from build123d import *

# Parameters (mm, degrees)
ESQUISSE1_R             = 16
BOSS_EXTRU_2_DEPTH      = 30
ESQUISSE2_R             = 18.5
BOSS_EXTRU_3_DEPTH      = 25
ESQUISSE3_R             = 1
ENL_V_MAT_EXTRU_1_DEPTH = 3.5
ESQUISSE5_R             = 6
BOSS_EXTRU_4_DEPTH      = 6
ESQUISSE6_R             = 3
BOSS_EXTRU_5_DEPTH      = 15.5
ESQUISSE7_W             = 7.308646468
ESQUISSE7_H             = 1
ENL_V_MAT_EXTRU_2_DEPTH = 12


with BuildPart() as part:
    # Esquisse1 → Boss.-Extru.2 (new body)
    with BuildSketch(Plane.XY):
        Circle(ESQUISSE1_R)
    extrude(amount=BOSS_EXTRU_2_DEPTH)

    # Esquisse2 → Boss.-Extru.3 (add)
    with BuildSketch(Plane.XY.offset(30)):
        Circle(ESQUISSE2_R)
    extrude(amount=BOSS_EXTRU_3_DEPTH)

    # Esquisse3 → Enlèv. mat.-Extru.1 (cut)
    with BuildSketch(Plane.XY.offset(55)):
        with Locations(Location((-15.5, 0, 0), (0, 0, 180))):
            Circle(ESQUISSE3_R)
        with Locations(Location((7.75, -13.423393759, 0), (0, 0, 180))):
            Circle(ESQUISSE3_R)
        with Locations(Location((15.5, 0, 0), (0, 0, 180))):
            Circle(ESQUISSE3_R)
        with Locations(Location((7.75, 13.423393759, 0), (0, 0, 180))):
            Circle(ESQUISSE3_R)
    extrude(amount=-ENL_V_MAT_EXTRU_1_DEPTH, mode=Mode.SUBTRACT)

    # Esquisse5 → Boss.-Extru.4 (add)
    with BuildSketch(Plane.XY.offset(55)):
        with Locations((0, 7)):
            Circle(ESQUISSE5_R)
    extrude(amount=BOSS_EXTRU_4_DEPTH)

    # Esquisse6 → Boss.-Extru.5 (add)
    with BuildSketch(Plane.XY.offset(61)):
        with Locations((0, 7)):
            Circle(ESQUISSE6_R)
    extrude(amount=BOSS_EXTRU_5_DEPTH)

    # Esquisse7 → Enlèv. mat.-Extru.2 (cut)
    with BuildSketch(Plane.XY.offset(76.5)):
        with Locations((0, 10)):
            Rectangle(ESQUISSE7_W, ESQUISSE7_H)
    extrude(amount=-ENL_V_MAT_EXTRU_2_DEPTH, mode=Mode.SUBTRACT)


solid = part.part
The model under review builds one solid part; all positions refer to its coordinate system, in mm. A direction names the side the tool comes from. Give positions to 0.01 mm unless a question says otherwise; leave off trailing zeros. Write each loop counter-clockwise with the first axis right and the second up, starting at its lowest first coordinate (ties: lowest second). Pieces come first, ordered by that corner, then holes.
1. Draft analysis for pull direction Y (two halves, no side actions). For faces 1 (the cylindrical face through (-3.47, -15.62, 14.79)), 2 (the flat face through (0, 0, 55)), 3 (the cylindrical face through (7.88, 12.43, 53.27)), state which applies: +Y half, -Y half, draft (parallel to the pull), parting line (faces both ways), or undercut.
2. For P1, Ø2, axis at x = 15, y = -0.5, coming from the +Z side; P2, Ø1.5, axis at x = -4, z = 37, coming from the -Y side; P3, Ø1, axis at y = 1, z = 53.5, coming from the +X side, all flat-tipped, find the tip position at first contact; note any pin that passes through.
3. Add section C-C, the plane z = 60. Write out the cut boundary in (x, y), plus the area to 3 significant figures.
4. Tool access review of faces 4 (the flat face through (0, 0, 0)), 5 (the flat face through (0, 9.5, 71)), 6 (the flat face through (-6, 15, 30)), 7 (the cylindrical face through (-4.01, -18.06, 42.32)), 8 (the cylindrical face through (-0.65, 4.07, 68.64)): name each direction out of +Z, -Z, +X, -X, +Y, -Y from which nothing blocks a thin tool from reaching the whole face with its end or side.
5. Add section B-B, the plane y = 0. Write out the cut boundary in (x, z), plus the area to 3 significant figures.
6. Wall thickness on L1, parallel to Y at x = 7.75, z = 52.4; L2, parallel to Z at x = 9, y = -14; L3, parallel to Y at x = 7, z = 53: over which ranges is each line inside the solid? List them lowest first.
7. Add section A-A, the plane x = 0. Write out the cut boundary in (y, z).
8. Add section D-D, the plane y = -9. Write out the cut boundary in (x, z).
Worked answers:
1. face 1: parting line
1. face 2: draft
1. face 3: undercut
2. P1: stops at z = 55
2. P2: stops at y = -18.21
2. P3: stops at x = 18.49
3. outline: circle Ø12 at (0, 7)
3. area: 113 mm2
4. face 4: -Z, +X, -X, +Y, -Y
4. face 5: +Z, +X, -X, +Y
4. face 6: -Z
4. face 7: +Z, -Z
4. face 8: +Z
5. outline: (-18.5, 30) - (-16, 30) - (-16, 0) - (16, 0) - (16, 30) - (18.5, 30) - (18.5, 55) - (16.5, 55) - (16.5, 51.5) - (14.5, 51.5) - (14.5, 55) - (-14.5, 55) - (-14.5, 51.5) - (-16.5, 51.5) - (-16.5, 55) - (-18.5, 55) - close
5. area: 1,870 mm2
6. L1: y = -16.8 to -14.42, -12.42 to 12.42, 14.42 to 16.8
6. L2: z = 30 to 55
6. L3: y = -17.12 to -14.08, -12.76 to 12.76, 14.08 to 17.12
7. outline: (-18.5, 30) - (-16, 30) - (-16, 0) - (16, 0) - (16, 30) - (18.5, 30) - (18.5, 55) - (13, 55) - (13, 61) - (10, 61) - (10, 64.5) - (9.5, 64.5) - (9.5, 76.5) - (4, 76.5) - (4, 61) - (1, 61) - (1, 55) - (-18.5, 55) - close
8. outline: (-16.16, 30) - (-13.23, 30) - (-13.23, 0) - (13.23, 0) - (13.23, 30) - (16.16, 30) - (16.16, 55) - (-16.16, 55) - close
